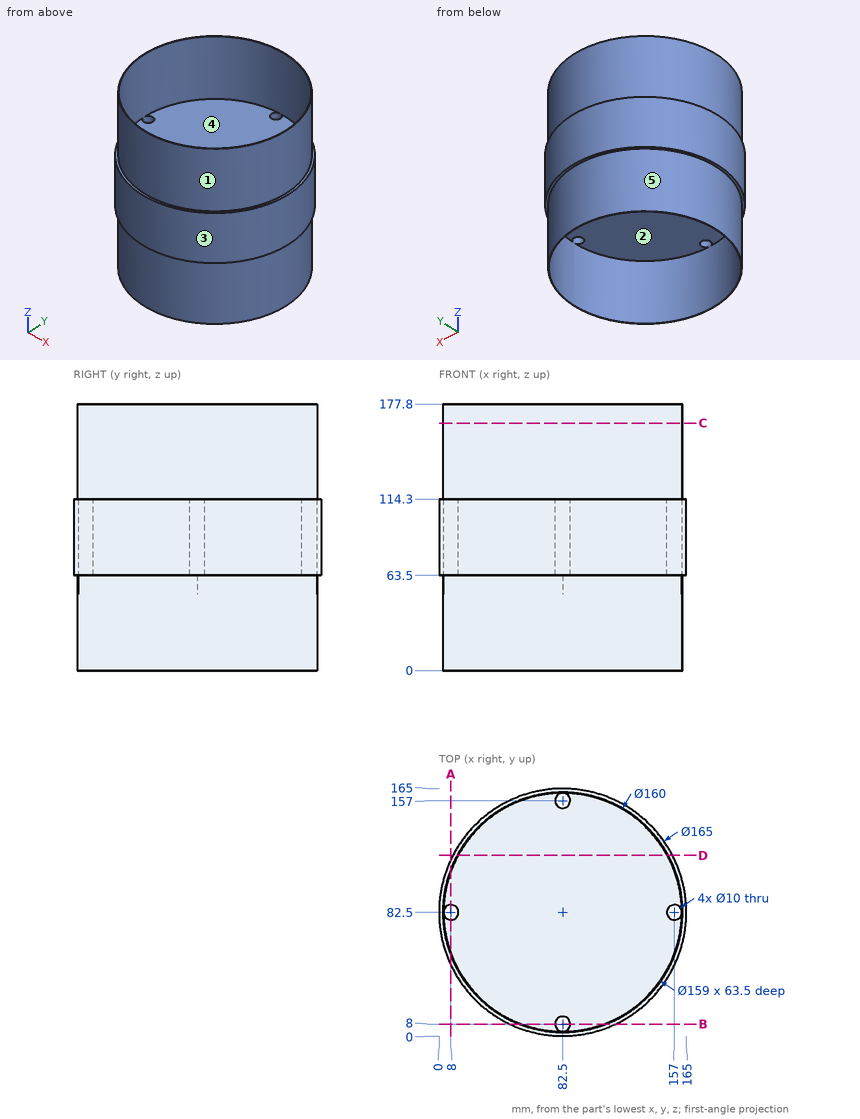
Design review of the part shown in the three views and the two pictorial views. Dimensions are in mm from the part's minimum x, y and z. A direction names the side the tool comes from. Give positions to 0.01 mm unless a question says otherwise; leave off trailing zeros. Loops run counter-clockwise (first coordinate to the right, second up) from the corner with the lowest first, then second, coordinate; pieces in that order, holes last. Notation, with made-up numbers: M -14.5,22.5 L 38.5,22.5 A13 ccw 38.5,39.5 Z; hole C 85.25,-7 d3. An arc over 180 degrees is marked long. Put each result on its own line as item: value. Start each with the question number.
(1) Machinability: for the marked faces 3, 4 and 5, which of the approach directions +Z, -Z, +X, -X, +Y, -Y give a long, thin tool a straight path to every point of the face, cutting with its end or side? Answer none if there is none.
(2) Add section D-D, the plane y = 120.5. Write out the cut boundary in (x, z).
(3) The part is to be moulded in two halves that separate along X. For the marked faces 1 and 2, say which applies: +X half, -X half, draft (parallel to the pull), parting line (faces both ways), or undercut.
(4) Wall thickness on L1, parallel to X at y = 82, z = 96; L2, parallel to X at y = 86, z = 100: over which ranges is each line inside the solid? List them lowest first.
(5) Add section C-C, the plane z = 165. Write out the cut boundary in (x, y), then the cut area to 3 significant figures.
(6) Add section A-A, the plane x = 8. Write out the cut boundary in (y, z).
(7) For pin 1 (16 mm diameter, centred on x = 157, y = 82.5, fed in from +Z); pin 2 (1.5 mm diameter, centred on x = 128, z = 94, fed in from -Y); pin 3 (1 mm diameter, centred on x = 105.5, z = 157.5, fed in from +Y); pin 4 (9 mm diameter, centred on x = 8, y = 82.5, fed in from -Z), all flat-tipped, find the tip position at first contact; note any pin that passes through.
Result:
1. face 3: +Z, -Z
1. face 4: +Z
1. face 5: -Z
2. outline: M 9.27,63.5 L 12.1,63.5 L 12.1,0 L 12.67,0 L 12.67,63.5 L 152.33,63.5 L 152.33,0 L 152.9,0 L 152.9,63.5 L 155.73,63.5 L 155.73,114.3 L 152.9,114.3 L 152.9,177.8 L 152.33,177.8 L 152.33,114.3 L 12.67,114.3 L 12.67,177.8 L 12.1,177.8 L 12.1,114.3 L 9.27,114.3 Z
3. face 1: parting line
3. face 2: undercut
4. L1: x = 0 to 3.03, 12.97 to 152.03, 161.97 to 165
4. L2: x = 0.07 to 4.43, 11.57 to 153.43, 160.57 to 164.93
5. outline: C 82.5,82.5 d160; hole C 82.5,82.5 d159
5. area: 251 mm^2
6. outline: M 47.06,63.5 L 53.35,63.5 L 53.35,0 L 54.75,0 L 54.75,63.5 L 77.5,63.5 L 77.5,114.3 L 54.75,114.3 L 54.75,177.8 L 53.35,177.8 L 53.35,114.3 L 47.06,114.3 Z; M 87.5,63.5 L 110.25,63.5 L 110.25,0 L 111.65,0 L 111.65,63.5 L 117.94,63.5 L 117.94,114.3 L 111.65,114.3 L 111.65,177.8 L 110.25,177.8 L 110.25,114.3 L 87.5,114.3 Z
7. pin 1: stops at z = 177.8
7. pin 2: stops at y = 13.19
7. pin 3: stops at y = 159.27
7. pin 4: passes through
